from build123d import *

# Parameters (mm, degrees)
EXTRUDE_1_DEPTH          = 5
SKETCH_3_W               = 20
SKETCH_3_H               = 20
EXTRUDE_2_DEPTH          = 5
SKETCH_4_R               = 1.75
CUT_EXTRUDE_1_DEPTH      = 6
CUT_EXTRUDE_2_DEPTH      = 1
CUT_EXTRUDE_2_DEPTH_BACK = 26
SKETCH_6_R               = 2.5
CUT_EXTRUDE_3_DEPTH      = 6


with BuildPart() as part:
    # ｽｹｯﾁ1 → ﾎﾞｽ - 押し出し1 (new body)
    with BuildSketch(Plane.XY):
        Polygon((-15, 10), (15, 10), (15, 0), (35, 0), (35, 50), (-35, 50), (-35, 0), (-15, 0), align=None)
    extrude(amount=EXTRUDE_1_DEPTH)

    # ｽｹｯﾁ3 → ﾎﾞｽ - 押し出し2 (add)
    with BuildSketch(Plane(origin=(0, 0, 0), x_dir=(1, 0, 0), z_dir=(0, 1, 0))):
        with Locations((-25, 10)):
            Rectangle(SKETCH_3_W, SKETCH_3_H)
        with Locations((25, 10)):
            Rectangle(SKETCH_3_W, SKETCH_3_H)
    extrude(amount=EXTRUDE_2_DEPTH)

    # ｽｹｯﾁ4 → ｶｯﾄ - 押し出し1 (cut, through all)
    with BuildSketch(Plane(origin=(0, 5, 0), x_dir=(1, 0, 0), z_dir=(0, 1, 0))):
        with Locations((-30, 5)):
            Circle(SKETCH_4_R)
        with Locations((-20, 15)):
            Circle(SKETCH_4_R)
        with Locations((20, 15)):
            Circle(SKETCH_4_R)
        with Locations((30, 5)):
            Circle(SKETCH_4_R)
    extrude(amount=-CUT_EXTRUDE_1_DEPTH, mode=Mode.SUBTRACT)

    # ｽｹｯﾁ5 → ｶｯﾄ - 押し出し2 (cut, two sides)
    with BuildSketch(Plane.XY.offset(5)) as cut_extrude_2_sk:
        Polygon((15, 50), (35, 30), (35, 50), align=None)
        Polygon((-35, 30), (-15, 50), (-35, 50), align=None)
    extrude(amount=CUT_EXTRUDE_2_DEPTH, mode=Mode.SUBTRACT)
    extrude(cut_extrude_2_sk.sketch, amount=-CUT_EXTRUDE_2_DEPTH_BACK, mode=Mode.SUBTRACT)

    # ｽｹｯﾁ6 → ｶｯﾄ - 押し出し3 (cut, through all)
    with BuildSketch(Plane(origin=(0, 0, 0), x_dir=(-1, 0, 0), z_dir=(0, 0, -1))):
        with Locations((-22, 30)):
            Circle(SKETCH_6_R)
        with Locations((0, 30)):
            Circle(SKETCH_6_R)
        with Locations((-10, 45)):
            Circle(SKETCH_6_R)
        with Locations((10, 45)):
            Circle(SKETCH_6_R)
        with Locations((22, 30)):
            Circle(SKETCH_6_R)
    extrude(amount=-CUT_EXTRUDE_3_DEPTH, mode=Mode.SUBTRACT)


solid = part.part
Build history of the part. All positions in model axes, mm. A direction names the side the tool comes from. Round coordinates to 2 decimals unless told otherwise and drop trailing zeros. Write each loop counter-clockwise with the first axis right and the second up, starting at its lowest first coordinate (ties: lowest second). Pieces come first, ordered by that corner, then holes. Notation, with made-up numbers: (5, 70.5) - (20, 70.5) arc R28 ccw to (20, 107.5) - close; hole circle Ø3 at (-27, 6). An arc over 180 degrees is marked (long way). One line per question, with ' | ' between items.
1. Band-saw the part on A-A, the plane x = -30. Write the cut outline in (y, z).
Results are:
outline: (0, -20) - (5, -20) - (5, -6.75) - (0, -6.75) - close; (0, -3.25) - (5, -3.25) - (5, 0) - (35, 0) - (35, 5) - (0, 5) - close
2. Mould opens along Y. For faces 4 (the face through (-25, 40, 3)), 5 (the face through (28.25, 2.54, -5.08)), 6 (the face through (23.84, 31.69, 2.46)), 7 (the face through (-9.46, 42.56, 2.46)) say: released by +Y, released by -Y, zero draft, split by the parting line, or undercut.
Results are:
face 4: released by +Y | face 5: zero draft | face 6: undercut | face 7: undercut
3. Band-saw the part on C-C, the plane z = -10.5. Write the cut outline in (x, y), and give its area (3 significant figures).
Results are:
outline: (-35, 0) - (-15, 0) - (-15, 5) - (-35, 5) - close; (15, 0) - (35, 0) - (35, 5) - (15, 5) - close | area: 200 mm^2
4. Drill centre lines: line 1 along Y through (x, z) = (0, 2.6); line 2 along Z through (x, y) = (30, 1); line 3 along X through (y, z) = (43, 1). Where is each one in solid material? Low to high. Write a range as from..to.
Results are:
line 1: 10..27.5, 32.5..50 | line 2: -20..-6.75, -3.25..5 | line 3: -22..-11.5, -8.5..8.5, 11.5..22
5. Drop flat-ended pins along their axis: pin 1 Ø6 at (x, y) = (5.5, 29.5) entering from -Z; pin 2 Ø6 at (x, z) = (24, -6.5) entering from +Y; pin 3 Ø6 at (y, z) = (44, -4) entering from -X; pin 4 Ø1.5 at (x, z) = (7, 1.5) entering from -Y. Give the stop position or say it passes through.
Results are:
pin 1: z = 0 | pin 2: y = 5 | pin 3: through | pin 4: y = 10
6. Band-saw the part on B-B, the plane z = -15. Write the cut outline in (x, y), and give its area (3 significant figures).
Results are:
outline: (-35, 0) - (-21.75, 0) - (-21.75, 5) - (-35, 5) - close; (-18.25, 0) - (-15, 0) - (-15, 5) - (-18.25, 5) - close; (15, 0) - (18.25, 0) - (18.25, 5) - (15, 5) - close; (21.75, 0) - (35, 0) - (35, 5) - (21.75, 5) - close | area: 165 mm^2
7. Tool access for faces 1 (the face through (25, 5, -10)), 2 (the face through (0, 25, 5)), 3 (the face through (0, 10, 2)): list every direction of +Z, -Z, +X, -X, +Y, -Y with a clear straight run to the whole face (end or side of a thin tool).
Results are:
face 1: -Z, +X, -X, +Y | face 2: +Z, +X, -X, +Y, -Y | face 3: +Z, -Z, -Y
8. Band-saw the part on D-D, the plane x = 11. Write the cut outline in (y, z).
Results are:
outline: (10, 0) - (42.71, 0) - (42.71, 5) - (10, 5) - close; (47.29, 0) - (50, 0) - (50, 5) - (47.29, 5) - close
